```python
from build123d import *

# Parameters (mm, degrees)
F1_DEPTH = 5
F3_R     = 26.5
F3_R_2   = 26
F6_DEPTH = 4


with BuildPart() as f1:
    # F0 (on Top) → F1 (new body)
    with BuildSketch(Plane.XY):
        with BuildLine():
            ThreePointArc((-14.25, 0), (0, 14.25), (14.25, 0))
            Line((14.25, 0), (15.25, 0))
            ThreePointArc((15.25, 0), (0, 15.25), (-15.25, 0))
            Line((-15.25, 0), (-14.25, 0))
        make_face()
        with BuildLine():
            Line((15.25, 0), (14.25, 0))
            ThreePointArc((14.25, 0), (0, -14.25), (-14.25, 0))
            Line((-14.25, 0), (-15.25, 0))
            ThreePointArc((-15.25, 0), (0, -15.25), (15.25, 0))
        make_face()
    extrude(amount=F1_DEPTH)

    # F4 (on Front) → F5 (revolve)
    with BuildSketch(Plane.XZ):
        Polygon((-26.5, 17), (-15.25, 5), (-14.25, 5), (-26, 17), align=None)
    revolve(axis=Axis((0, 0, 35.630243), (0, 0, 1)))

    # F3 (on offset) → F6 (join)
    with BuildSketch(Plane.XY.offset(17)):
        Circle(F3_R)
        Circle(F3_R_2, mode=Mode.SUBTRACT)
    extrude(amount=F6_DEPTH)


solid = f1.part
```
Design review of the part built by this model. Coordinates are the model's own, in mm. A direction names the side the tool comes from. Coordinates: 2 decimals unless noted, no trailing zeros. Write each loop counter-clockwise with the first axis right and the second up, starting at its lowest first coordinate (ties: lowest second). Pieces come first, ordered by that corner, then holes.
1) Mouldability with a two-part tool opening along Y and no side actions: class faces 1 (the flat face through (-5, 14, 0)), 2 (the cylindrical face through (-3.09, 13.91, 2.46)), 3 (the conical face through (12.535, 9.612, 5.583)), 4 (the conical face through (-6.915, 13.294, 5.751)) as +Y half, -Y half, draft (parallel to the pull), parting line (faces both ways), or undercut.
2) Add section A-A (y = 0). Write out the cut boundary in (x, z), plus the area to 3 significant figures.
3) To check wall thickness, follow L1, parallel to Y at x = 0, z = 17.95; L2, parallel to Y at x = 0, z = 1.1. State the ranges of each line that lie inside material, in increasing order.
4) Insertion check: pin 1 (3 mm diameter, centred on x = 10.5, z = 11.5, fed in from +Y); pin 2 (1 mm diameter, centred on y = -8.5, z = 11, fed in from -X); pin 3 (6 mm diameter, centred on x = -16, y = 11.5, fed in from +Z); pin 4 (23 mm diameter, centred on x = 0, y = 0, fed in from -Z). Each pin has a flat end and moves straight along its axis. Give the tip position at first contact, or say it passes through.
5) Machinability: for faces 5 (the cylindrical face through (3.306, 14.887, 2.465)), 6 (the cylindrical face through (-20.633, -15.821, 18.972)), 7 (the flat face through (19.5, -17.5, 21)), which of the approach directions +Z, -Z, +X, -X, +Y, -Y give a long, thin tool a straight path to every point of the face, cutting with its end or side? Answer none if there is none.
6) Add section C-C (z = 2.25). Write out the cut boundary in (x, y), plus the area to 3 significant figures.
7) Add section D-D (z = 7.5). Write out the cut boundary in (x, y).
Check result:
1. face 1: draft
1. face 2: undercut
1. face 3: parting line
1. face 4: undercut
2. outline: (-26.5, 17) - (-15.25, 5) - (-15.25, 0) - (-14.25, 0) - (-14.25, 5) - (-26, 17) - (-26, 21) - (-26.5, 21) - close; (14.25, 0) - (15.25, 0) - (15.25, 5) - (26.5, 17) - (26.5, 21) - (26, 21) - (26, 17) - (14.25, 5) - close
2. area: 32.0 mm2
3. L1: y = -26.5 to -26, 26 to 26.5
3. L2: y = -15.25 to -14.25, 14.25 to 15.25
4. pin 1: stops at y = 20.35
4. pin 2: stops at x = -19.62
4. pin 3: stops at z = 13.63
4. pin 4: passes through
5. face 5: -Z
5. face 6: +Z
5. face 7: +Z, +X, -X, +Y, -Y
6. outline: circle Ø30.5 at (0, 0); hole circle Ø28.5 at (0, 0)
6. area: 92.7 mm2
7. outline: circle Ø35.19 at (0, 0); hole circle Ø33.4 at (0, 0)
